Job drawing, mm, ordinate dimensions from the low corner. One solid piece. Give positions to 0.01 mm unless a question says otherwise; leave off trailing zeros. Order: outer loops, then holes, each group sorted by start corner. A loop starts at its lowest first (then second) coordinate and runs counter-clockwise, first axis right, second up. Notation, with made-up numbers: (49, 75.25) -> (96, 75.25) arc R27 ccw to (96, 109.25) -> close; hole circle Ø4 at (-8.75, -22.75). An arc over 180 degrees is marked (long way). Use CSV: the item, a comma, the result in double quotes. Start each with the question number.
1. Wall check: line 1 (Y direction, x = 11, z = 26); line 2 (Z direction, x = 7.75, y = 381) (3 decimals); line 3 (Y direction, x = 6.25, z = 27). Give the ranges that are in metal, low to high. Write a range as from..to.
2. Cut at B-B on y = 279.4. List the corners of the cut face in (x, z) (3 decimals), then the cut area to 3 significant figures.
3. Cut at C-C on x = 10.25. List the corners of the cut face in (y, z) (3 decimals), then the cut area to 3 significant figures.
4. Cut at A-A on z = 25.4. List the corners of the cut face in (x, y) (3 decimals), then the cut area to 3 significant figures.
5. Drop flat-ended pins along their axis: pin 1 (17 mm diameter, centred on y = 279.4, z = 25.4, fed in from +X); pin 2 (1 mm diameter, centred on x = 9, z = 40.5, fed in from -Y). Give the stop position or say it passes through.
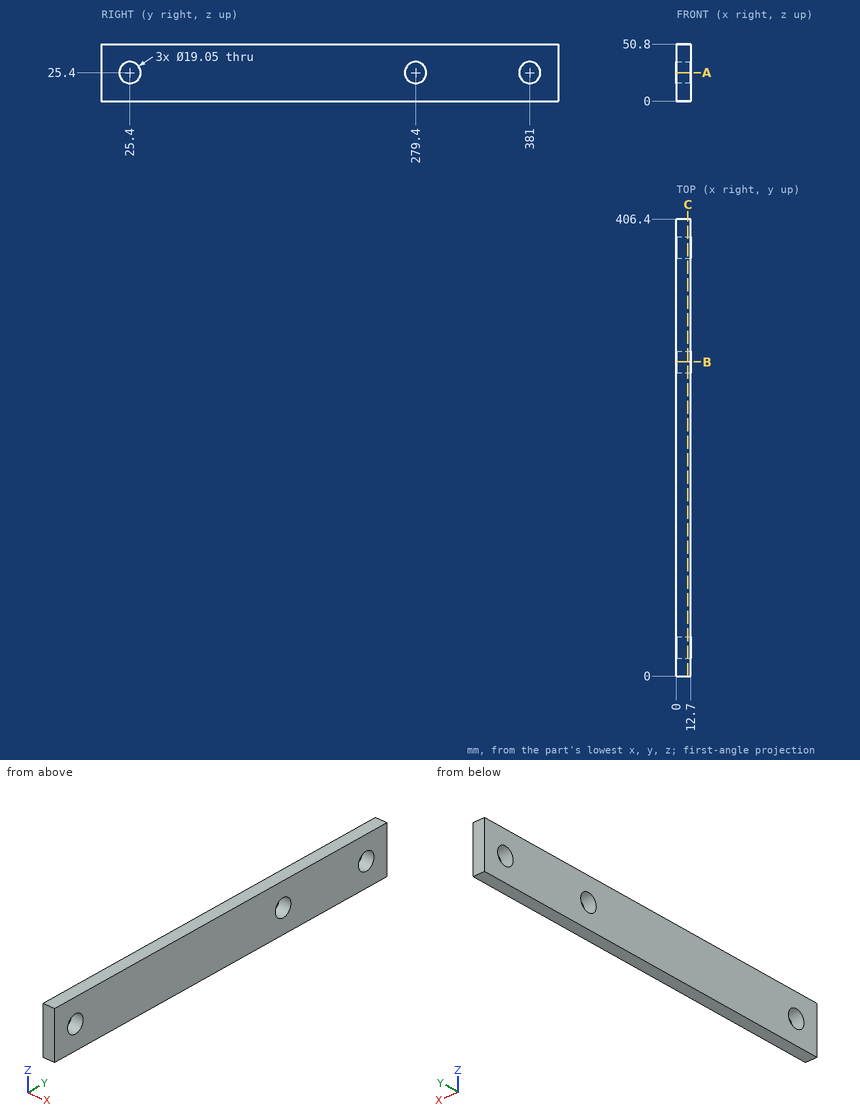
Verdict:
1,line 1,"0..15.89, 34.91..269.89, 288.91..371.49, 390.51..406.4"
1,line 2,"0..15.875, 34.925..50.8"
1,line 3,"0..16.01, 34.79..270.01, 288.79..371.61, 390.39..406.4"
2,outline,"(0, 0) -> (12.7, 0) -> (12.7, 15.875) -> (0, 15.875) -> close; (0, 34.925) -> (12.7, 34.925) -> (12.7, 50.8) -> (0, 50.8) -> close"
2,area,"403 mm^2"
3,outline,"(0, 0) -> (406.4, 0) -> (406.4, 50.8) -> (0, 50.8) -> close; hole circle Ø19.05 at (25.4, 25.4); hole circle Ø19.05 at (279.4, 25.4); hole circle Ø19.05 at (381, 25.4)"
3,area,"19,800 mm^2"
4,outline,"(0, 0) -> (12.7, 0) -> (12.7, 15.875) -> (0, 15.875) -> close; (0, 34.925) -> (12.7, 34.925) -> (12.7, 269.875) -> (0, 269.875) -> close; (0, 288.925) -> (12.7, 288.925) -> (12.7, 371.475) -> (0, 371.475) -> close; (0, 390.525) -> (12.7, 390.525) -> (12.7, 406.4) -> (0, 406.4) -> close"
4,area,"4,440 mm^2"
5,pin 1,"through"
5,pin 2,"y = 0"
